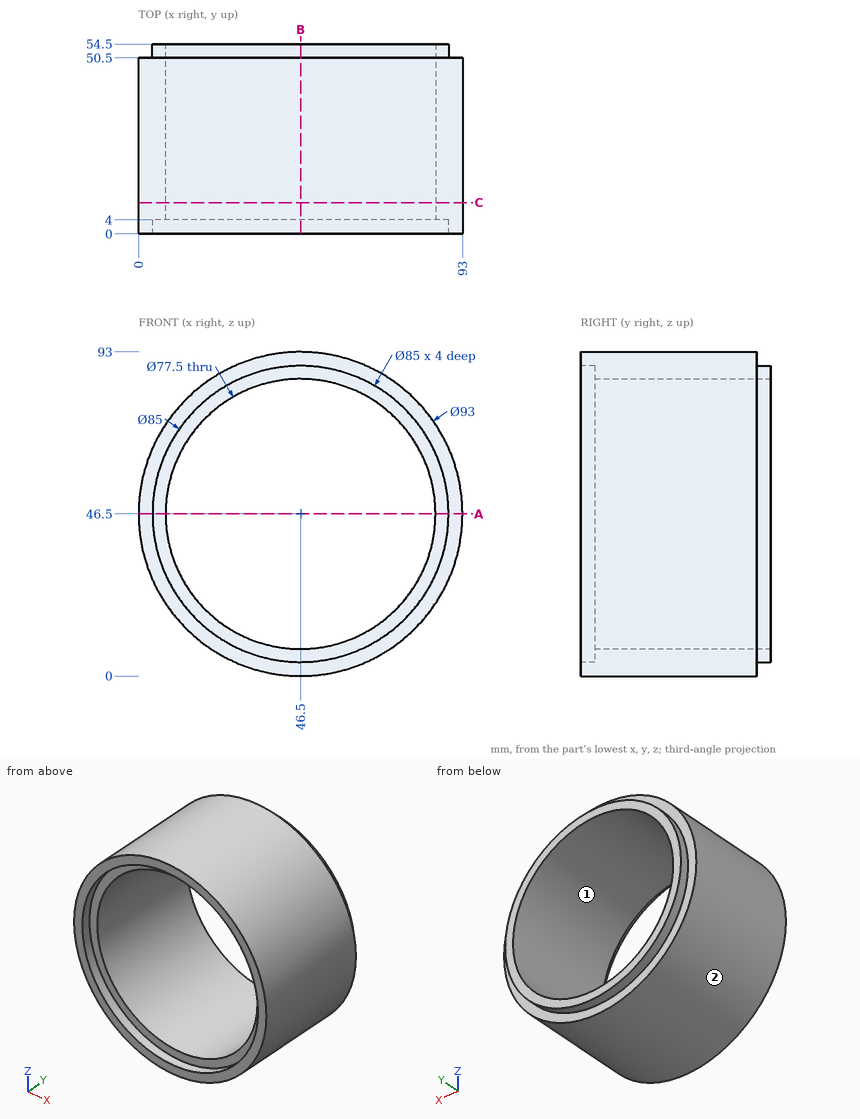
Design review of the part shown in the three views and the two pictorial views. Dimensions are in mm from the part's minimum x, y and z. Round coordinates to 2 decimals unless told otherwise and drop trailing zeros. Loops run counter-clockwise (first coordinate to the right, second up) from the corner with the lowest first, then second, coordinate; pieces in that order, holes last. Notation, with made-up numbers: (-1, 28.25) - (43, 28.25) arc R4 ccw to (43, 33.25) - close; hole circle Ø6 at (-40, 84). An arc over 180 degrees is marked (long way). One line per item, written item: value. Start each with the question number.
Item 1: Take a section at B-B (x = 46.5). Give the boundary of the cut face in (y, z), plus the area to 3 significant figures.
Item 2: Take a section at C-C (y = 9). Give the boundary of the cut face in (x, z).
Item 3: Take a section at A-A (z = 46.5). Give the boundary of the cut face in (x, y).
Item 4: Clearance check with flat-ended pins moving along their axes: pin 1 Ø12 at (x, y) = (63, 18.5) entering from -Z; pin 2 Ø6 at (y, z) = (43.5, 28) entering from -X; pin 3 Ø12 at (y, z) = (33.5, 22.5) entering from +X. State where each tip first meets the part, or that it passes through.
Item 5: For L1, parallel to Z at x = 46, y = 44; L2, parallel to Z at x = 46.5, y = 0.95; L3, parallel to X at y = 17, z = 65.5, list the stretches that pass through material, from the lowest coordinate up.
Item 6: The part is to be moulded in two halves that separate along Z. For the marked faces 1 and 2, say which applies: +Z half, -Z half, draft (parallel to the pull), parting line (faces both ways), or undercut.
Answer below:
1. outline: (0, 0) - (50.5, 0) - (50.5, 4) - (54.5, 4) - (54.5, 7.75) - (4, 7.75) - (4, 4) - (0, 4) - close; (0, 89) - (4, 89) - (4, 85.25) - (54.5, 85.25) - (54.5, 89) - (50.5, 89) - (50.5, 93) - (0, 93) - close
1. area: 783 mm2
2. outline: circle Ø93 at (46.5, 46.5); hole circle Ø77.5 at (46.5, 46.5)
3. outline: (0, 0) - (4, 0) - (4, 4) - (7.75, 4) - (7.75, 54.5) - (4, 54.5) - (4, 50.5) - (0, 50.5) - close; (85.25, 4) - (89, 4) - (89, 0) - (93, 0) - (93, 50.5) - (89, 50.5) - (89, 54.5) - (85.25, 54.5) - close
4. pin 1: stops at z = 1.2
4. pin 2: stops at x = 2.66
4. pin 3: stops at x = 89.37
5. L1: z = 0 to 7.75, 85.25 to 93
5. L2: z = 0 to 4, 89 to 93
5. L3: x = 4.06 to 12.73, 80.27 to 88.94
6. face 1: undercut
6. face 2: parting line
